Autodesk Inventor part; units mm, degrees
ref_plane "Work Plane1" through (-10, 0, 0) normal (1, 0, 0) x (0, 0, -1)
ref_plane "YZ Plane" through (0, 0, 0) normal (1, 0, 0) x (0, 1, 0)
ref_plane "XZ Plane" through (0, 0, 0) normal (0, 1, 0) x (-1, 0, 0)
sketch "Sketch1" plane through (0, 0, 0) normal (0, 1, 0) x (-1, 0, 0)
  circle A0 centre (0, 0) radius 10
  dimension "d0" = 20
extrude "Extrusion1" add sketch "Sketch1" along normal blind 7
sketch "Sketch2" plane through (0, 7, 0) normal (0, 1, 0) x (1, 0, 0)
  circle A0 centre (0, 0) radius 10
  arc A1 (0, -3) -> (0, 3) centre (0, 0) ccw
  line L0 (0, -3) -> (0, 3)
  dimension "d3" = 6
extrude "Extrusion2" cut sketch "Sketch2" against normal blind 4 contours L0 A1
sketch "Sketch3" plane through (0, 0, 0) normal (0, -1, 0) x (1, 0, 0)
  line L0 (0, 3) -> (0, -3)
  circle A0 centre (0, 0) radius 3
extrude "Extrusion3" cut sketch "Sketch3" against normal blind 1
ref_plane "Work Plane1" through (-10, 0, 0) normal (1, 0, 0) x (0, 0, -1)
sketch "Sketch4" plane through (-10, 0, 0) normal (1, 0, 0) x (0, 0, -1)
  line L0 (10, 7) -> (-10, 7)
  circle A0 centre (0, 5) radius 1.125
  point P0 (0, 0)
  dimension "d9" = 2.25
extrude "Extrusion4" cut sketch "Sketch4" along normal up to surface (10 mm away)
sketch "Sketch5" plane through (0, 7, 0) normal (0, 1, 0) x (1, 0, 0)
  circle A0 centre (0, 0) radius 6.985
  line L0 (0, 0) -> (6.985, 0) construction
  circle A1 centre (-4.9391, 4.9391) radius 1.5
  circle A2 centre (-4.9391, -4.9391) radius 1.5
  circle A3 centre (4.9391, -4.9391) radius 1.5
  circle A4 centre (4.9391, 4.9391) radius 1.5
  dimension "d14" = 3
  dimension "d17" = 360
extrude "Extrusion5" cut sketch "Sketch5" against normal up to surface (7 mm away) contours A4 A0 | A0 A4 | A3 A0 | A0 A3 | A1 A0 | A0 A1 | A2 A0 | A0 A2
sketch "Sketch6" plane through (0, 7, 0) normal (0, 1, 0) x (1, 0, 0)
  circle A0 centre (0, 0) radius 10
  circle A1 centre (-4.9391, 4.9391) radius 1.5
  circle A2 centre (-4.9391, 4.9391) radius 1.5
  circle A3 centre (4.9391, 4.9391) radius 1.5
  circle A4 centre (4.9391, 4.9391) radius 1.5
  circle A5 centre (4.9391, -4.9391) radius 1.5
  circle A6 centre (4.9391, -4.9391) radius 1.5
  circle A7 centre (-4.9391, -4.9391) radius 1.5
  circle A8 centre (-4.9391, -4.9391) radius 1.5
  circle A9 centre (-4.9391, -4.9391) radius 2.075
  circle A10 centre (4.9391, -4.9391) radius 2.075
  circle A11 centre (4.9391, 4.9391) radius 2.075
  circle A12 centre (-4.9391, 4.9391) radius 2.075
  line L0 (0, -3) -> (0, 3)
  arc A13 (0, -3) -> (0, 3) centre (0, 0) ccw
  arc A14 (0, -3) -> (0, 3) centre (0, 0) ccw
  line L1 (0, -3) -> (0, 3)
  dimension "d21" = 4.15
extrude "Extrusion6" add sketch "Sketch6" along normal blind 4 contours A0
equation "\"d19\" = d14"
properties part number "Twist_Attachment_To_Servo_Horn"
Work out the finished part from the listing and answer in its coordinate system (mm). A direction names the side the tool comes from. Round coordinates to 2 decimals unless told otherwise and drop trailing zeros. Loops run counter-clockwise (first coordinate to the right, second up) from the corner with the lowest first, then second, coordinate; pieces in that order, holes last.
(1) The mould has two halves that part along Z. Classify faces 4 (the flat face through (-2.1, 0, 2.4)), 5 (the cylindrical face through (3, 7, 0)), 6 (the cylindrical face through (-5.389, 8.972, -6.965)): pulls with the +Z half, pulls with the -Z half, needs draft (parallel to the pull), parting line crosses it, or undercut.
Computed values:
face 4: needs draft
face 5: undercut
face 6: undercut
(2) The part is cut by section B-B, the plane x = -4.75. Give the vertices of the cut face in (y, z) (3 decimals).
Computed values:
outline: (0, -8.8) - (11, -8.8) - (11, -7.005) - (7, -7.005) - (7, -6.427) - (0, -6.427) - close; (0, -3.451) - (7, -3.451) - (7, -2.873) - (11, -2.873) - (11, 2.873) - (7, 2.873) - (7, 3.451) - (0, 3.451) - close; (0, 6.427) - (7, 6.427) - (7, 7.005) - (11, 7.005) - (11, 8.8) - (0, 8.8) - close; hole circle Ø2.25 at (5, 0)
(3) The part is cut by section C-C, the plane y = 5. Give the vertices of the cut face in (x, z) (3 decimals).
Computed values:
outline: (-9.937, -1.125) arc R10 ccw (long way) to (-9.937, 1.125) - (0, 1.125) - (0, 3) arc R3 cw to (0, -3) - (0, -1.125) - close; hole circle Ø3 at (-4.939, -4.939); hole circle Ø3 at (-4.939, 4.939); hole circle Ø3 at (4.939, -4.939); hole circle Ø3 at (4.939, 4.939)
(4) The part is cut by section A-A, the plane z = 0. Give the vertices of the cut face in (x, y) (3 decimals).
Computed values:
outline: (-10, 0) - (-3, 0) - (-3, 1) - (3, 1) - (3, 0) - (10, 0) - (10, 11) - (3, 11) - (3, 3) - (0, 3) - (0, 3.875) - (-10, 3.875) - close; (-10, 6.125) - (0, 6.125) - (0, 11) - (-10, 11) - close
(5) For faces 1 (the cylindrical face through (4.614, 3.549, -3.475)), 2 (the cylindrical face through (6.05, 8.97, 6.69)), 3 (the flat face through (0, 1, 0)), determine the directions among +Z, -Z, +X, -X, +Y, -Y from which every point of the face is accessible in a straight line to the end or side of a thin tool.
Computed values:
face 1: +Y, -Y
face 2: +Y
face 3: -Y
(6) Each of these flat-tipped pins is pushed along its axis until it touches: P1, Ø3, axis at x = -4, y = 9.5, coming from the +Z side; P2, Ø4, axis at x = 7, y = 2, coming from the -Z side; P3, Ø1.5, axis at y = 7, z = -7.5, coming from the -X side. Where does it stop, or does it pass through?
Computed values:
P1: stops at z = 9.68
P2: stops at z = -8.66
P3: stops at x = -7.38
(7) Find the intervals of material crossed by L1, parallel to Z at x = -4, y = 4.75; L2, parallel to Z at x = -4.75, y = 10; L3, parallel to X at y = 8, z = 3.25, in increasing order.
Computed values:
L1: z = -9.17 to -6.11, -3.77 to -1.1, 1.1 to 3.77, 6.11 to 9.17
L2: z = -8.8 to -7.01, -2.87 to 2.87, 7.01 to 8.8
L3: x = -9.46 to -6.14, -3.73 to 3.73, 6.14 to 9.46
(8) The part is cut by section D-D, the plane y = 3.25. Give the vertices of the cut face in (x, z).
Computed values:
outline: circle Ø20 at (0, 0); hole circle Ø3 at (-4.94, -4.94); hole circle Ø3 at (-4.94, 4.94); hole (0, -3) arc R3 ccw to (0, 3) - close; hole circle Ø3 at (4.94, -4.94); hole circle Ø3 at (4.94, 4.94)
